Build history of the part. All positions in model axes, mm. A direction names the side the tool comes from. Round coordinates to 2 decimals unless told otherwise and drop trailing zeros. Write each loop counter-clockwise with the first axis right and the second up, starting at its lowest first coordinate (ties: lowest second). Pieces come first, ordered by that corner, then holes. Notation, with made-up numbers: (55, 31) -> (69, 31) arc R27 ccw to (69, 60) -> close; hole circle Ø11 at (82, -35). An arc over 180 degrees is marked (long way). Answer in a Markdown table with one row per item.
```python
from build123d import *

# Parameters (mm, degrees)
BOSS_EXTRUDE1_DEPTH = 15
BOSS_EXTRUDE2_REACH = 24.564
SKETCH2_R           = 5
SKETCH13_R          = 2.5
CUT_EXTRUDE2_DEPTH  = 27.563859895
SKETCH14_R          = 3.35
BOSS_EXTRUDE4_DEPTH = 7.1
SKETCH15_R          = 1.8
CUT_EXTRUDE3_DEPTH  = 30.664386187


with BuildPart() as part:
    # Sketch1 → Boss-Extrude1 (new body, symmetric)
    with BuildSketch(Plane.XY):
        with BuildLine():
            Line((23.077088849, -19.363976742), (20.77895552, -17.435613913))
            ThreePointArc((20.77895552, -17.435613913), (0, -27.125), (-20.77895552, -17.435613913))
            Line((-20.77895552, -17.435613913), (-23.077088849, -19.363976742))
            ThreePointArc((-23.077088849, -19.363976742), (0, -30.125), (23.077088849, -19.363976742))
        make_face()
    extrude(amount=BOSS_EXTRUDE1_DEPTH, both=True)

    # Sketch2 → Boss-Extrude2 (add, up to next)
    with BuildSketch(Plane(origin=(0, -40, 0), x_dir=(1, 0, 0), z_dir=(0, 1, 0)), mode=Mode.PRIVATE) as boss_extrude2_sk1:
        Circle(SKETCH2_R)
    boss_extrude2_tool1 = extrude(boss_extrude2_sk1.sketch, amount=BOSS_EXTRUDE2_REACH, mode=Mode.PRIVATE) - part.part
    add(boss_extrude2_tool1.solids().sort_by_distance((0, -40, 0))[0])

    # Sketch13 → Cut-Extrude2 (cut, through all)
    with BuildSketch(Plane(origin=(15.0625, -26.089015289, 0), x_dir=(-0.866025404, -0.5, 0), z_dir=(0.5, -0.866025404, 0))):
        with Locations((0, 8)):
            Circle(SKETCH13_R)
        with Locations((0, -8)):
            Circle(SKETCH13_R)
    cut_extrude2 = extrude(amount=-CUT_EXTRUDE2_DEPTH, mode=Mode.SUBTRACT)

    # Mirror1: Cut-Extrude2 across plane
    add(cut_extrude2.mirror(Plane(origin=(0, 0, 0), x_dir=(0, 0, 1), z_dir=(1, 0, 0))), mode=Mode.SUBTRACT)

    # Sketch14 → Boss-Extrude4 (add)
    with BuildSketch(Plane.XZ.offset(40)):
        Circle(SKETCH14_R)
    extrude(amount=BOSS_EXTRUDE4_DEPTH)

    # Sketch15 → Cut-Extrude3 (cut, through all)
    with BuildSketch(Plane.XZ.offset(47.1)):
        Circle(SKETCH15_R)
    extrude(amount=-CUT_EXTRUDE3_DEPTH, mode=Mode.SUBTRACT)


solid = part.part
```
Q1. Saw through at B-B on z = 0. Write the cut outline in (x, y) (3 decimals).
A:
| item | result |
|---|---|
| outline | (-23.077, -19.364) arc R30.125 ccw to (-5, -29.707) -> (-5, -40) -> (-3.35, -40) -> (-3.35, -47.1) -> (-1.8, -47.1) -> (-1.8, -27.065) arc R27.125 cw to (-20.779, -17.436) -> close; (1.8, -47.1) -> (3.35, -47.1) -> (3.35, -40) -> (5, -40) -> (5, -29.707) arc R30.125 ccw to (23.077, -19.364) -> (20.779, -17.436) arc R27.125 cw to (1.8, -27.065) -> close |
Q2. Wall check: line 1 (X direction, y = -37, z = 0); line 2 (Z direction, x = 0, y = -42.25). Give the ranges that are in metal, low to high. Write a range as [from, to].
A:
| item | result |
|---|---|
| line 1 | [-5, -1.8], [1.8, 5] |
| line 2 | [-3.35, -1.8], [1.8, 3.35] |
Q3. Saw through at D-D on x = -18. Write the cut outline in (y, z), plus the area to 3 significant figures.
A:
| item | result |
|---|---|
| outline | (-24.16, -15) -> (-20.29, -15) -> (-20.29, 15) -> (-24.16, 15) -> close |
| area | 116 mm² |
Q4. Saw through at C-C on y = -20. Write the cut outline in (x, z), plus the area to 3 significant figures.
A:
| item | result |
|---|---|
| outline | (-22.53, -15) -> (-18.32, -15) -> (-18.32, 15) -> (-22.53, 15) -> close; (18.32, -15) -> (22.53, -15) -> (22.53, 15) -> (18.32, 15) -> close |
| area | 252 mm² |
Q5. Which spindle directions (+Z, -Z, +X, -X, +Y, -Y) get a long thin tool onto all of the face, cutting with end or side? Do faces 4 (the flat face through (-1.2, -40, 3.3)), 5 (the flat face through (0, -28, 15)). Say none if no direction does.
A:
| item | result |
|---|---|
| face 4 | -Y |
| face 5 | +Z, +X, -X, +Y, -Y |
Q6. Saw through at A-A on x = 0. Write the cut outline in (y, z) (3 decimals).
A:
| item | result |
|---|---|
| outline | (-47.1, -3.35) -> (-40, -3.35) -> (-40, -5) -> (-30.125, -5) -> (-30.125, -15) -> (-27.125, -15) -> (-27.125, -1.8) -> (-47.1, -1.8) -> close; (-47.1, 1.8) -> (-27.125, 1.8) -> (-27.125, 15) -> (-30.125, 15) -> (-30.125, 5) -> (-40, 5) -> (-40, 3.35) -> (-47.1, 3.35) -> close |
Q7. Two-plate mould, pull along Z, no slides. Class faces 1 (the cylindrical face through (-14.76, -24.49, 10.44)), 2 (the cylindrical face through (-1.08, -34.93, 4.88)), 3 (the flat face through (0, -28, -15)): released by +Z, released by -Z, zero draft, split by the parting line, or undercut.
A:
| item | result |
|---|---|
| face 1 | undercut |
| face 2 | split by the parting line |
| face 3 | released by -Z |
Q8. Drop flat-ended pins along their axis: P1, Ø4.5, axis at x = 0, z = 0, coming from the +Y side; P2, Ø6, axis at x = 14, z = 3, coming from the +Y side; P3, Ø5, axis at x = -17, z = -11.5, coming from the -Y side. Give the stop position or say it passes through.
A:
| item | result |
|---|---|
| P1 | y = -27.03 |
| P2 | y = -21.14 |
| P3 | y = -26.41 |
